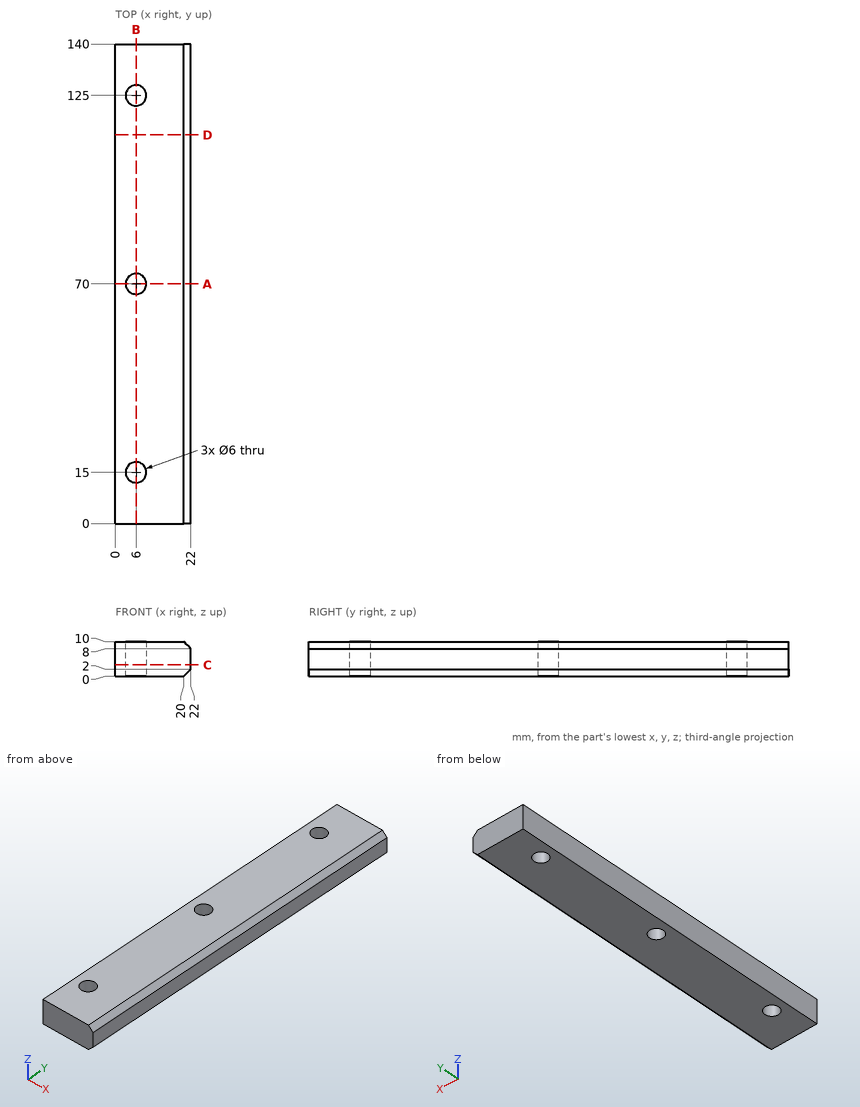
Here's the drawing with two shaded views (mm, measured from the low corner). I have some questions. Coordinates: 2 decimals unless noted, no trailing zeros. Write each loop counter-clockwise with the first axis right and the second up, starting at its lowest first coordinate (ties: lowest second). Pieces come first, ordered by that corner, then holes. Notation, with made-up numbers: (13.5, 44) - (24.5, 44) arc R33 cw to (24.5, 76) - close; hole circle Ø11 at (39, 9.25). An arc over 180 degrees is marked (long way). Return JSON: item names as keys, results as strings.
Q1. If we section it at B-B (x = 6): Please give me the cut outline in (y, z).
Computed values:
{"outline": "(0, 0) - (12, 0) - (12, 10) - (0, 10) - close; (18, 0) - (67, 0) - (67, 10) - (18, 10) - close; (73, 0) - (122, 0) - (122, 10) - (73, 10) - close; (128, 0) - (140, 0) - (140, 10) - (128, 10) - close"}
Q2. If we section it at C-C (z = 3.25): Please give me the cut outline in (x, y).
Computed values:
{"outline": "(0, 0) - (22, 0) - (22, 140) - (0, 140) - close; hole circle Ø6 at (6, 15); hole circle Ø6 at (6, 70); hole circle Ø6 at (6, 125)"}
Q3. If we section it at A-A (y = 70): Please give me the cut outline in (x, z), then the cut area to 3 significant figures.
Computed values:
{"outline": "(0, 0) - (3, 0) - (3, 10) - (0, 10) - close; (9, 0) - (20, 0) - (22, 2) - (22, 8) - (20, 10) - (9, 10) - close", "area": "156 mm2"}
Q4. Please list where these lines run through material, in increasing order: L1, parallel to Y at x = 6, z = 5.5; L2, parallel to Y at x = 8.75, z = 6.25; L3, parallel to X at y = 54, z = 0.75. Write a range as from..to.
Computed values:
{"L1": "y = 0..12, 18..67, 73..122, 128..140", "L2": "y = 0..13.8, 16.2..68.8, 71.2..123.8, 126.2..140", "L3": "x = 0..20.75"}
Q5. I'm going to push a flat-ended pin straight in: pin 1 Ø1 at (x, z) = (18.5, 7) entering from -Y. Where does the tip first touch, or does it pass through?
Computed values:
{"pin 1": "stops at y = 0"}
Q6. If we section it at D-D (y = 113.5): Please give me the cut outline in (x, z).
Computed values:
{"outline": "(0, 0) - (20, 0) - (22, 2) - (22, 8) - (20, 10) - (0, 10) - close"}
